Geometry: see drawing. Coordinates: mm, zero at the bounding-box minimum. Round coordinates to 2 decimals unless told otherwise and drop trailing zeros. Write each loop counter-clockwise with the first axis right and the second up, starting at its lowest first coordinate (ties: lowest second). Pieces come first, ordered by that corner, then holes. Notation, with made-up numbers: (78, 22.25) -> (123, 22.25) arc R13 cw to (123, 26.25) -> close; hole circle Ø4 at (-6, 7). An arc over 180 degrees is marked (long way). Write item = value, one per line.
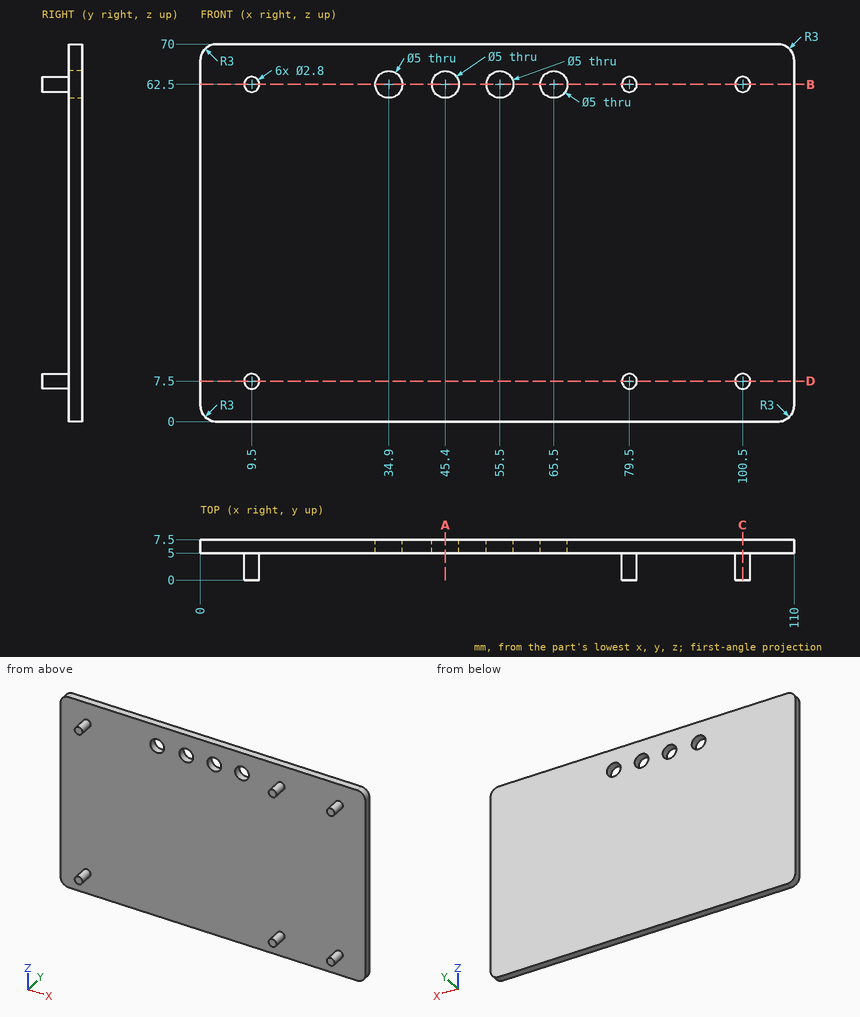
1) Cut plane A-A (x = 45.4). Return the cut outline in (y, z), and give its area (4 significant figures).
Solutions:
outline = (5, 0) -> (7.5, 0) -> (7.5, 60) -> (5, 60) -> close; (5, 65) -> (7.5, 65) -> (7.5, 70) -> (5, 70) -> close
area = 162.5 mm^2
2) First-contact query: P1, Ø4, axis at x = 35.5, z = 15.5, coming from the -Y side; P2, Ø4.5, axis at x = 65.5, z = 62.5, coming from the -Y side. Flat tips, straight axial feed; report the tip coordinate or a pass-through.
Solutions:
P1 = 5
P2 = through
3) Cut plane D-D (z = 7.5). Return the cut outline in (x, y), and give its area (3 significant figures).
Solutions:
outline = (0, 5) -> (8.1, 5) -> (8.1, 0) -> (10.9, 0) -> (10.9, 5) -> (78.1, 5) -> (78.1, 0) -> (80.9, 0) -> (80.9, 5) -> (99.1, 5) -> (99.1, 0) -> (101.9, 0) -> (101.9, 5) -> (110, 5) -> (110, 7.5) -> (0, 7.5) -> close
area = 317 mm^2
4) Line query: L1, parallel to X at y = 5.55, z = 62.5; L2, parallel to Z at x = 65.5, y = 6.4; L3, parallel to Y at x = 72, z = 58. Output: solid intervals per line, ascending. Write a range as from..to.
Solutions:
L1 = 0..32.4, 37.4..42.9, 47.9..53, 58..63, 68..110
L2 = 0..60, 65..70
L3 = 5..7.5
5) Cut plane C-C (x = 100.5). Return the cut outline in (y, z).
Solutions:
outline = (0, 6.1) -> (5, 6.1) -> (5, 0) -> (7.5, 0) -> (7.5, 70) -> (5, 70) -> (5, 63.9) -> (0, 63.9) -> (0, 61.1) -> (5, 61.1) -> (5, 8.9) -> (0, 8.9) -> close
6) Cut plane B-B (z = 62.5). Count the separate pieces of the cut face and the enclosed holes in it, and give its area (3 significant figures).
Solutions:
separate_pieces = 5
enclosed_holes = 0
area = 267 mm^2
